Could you check a few things on this model? Use its own coordinates, in mm. Round coordinates to 2 decimals unless told otherwise and drop trailing zeros. Loops run counter-clockwise (first coordinate to the right, second up) from the corner with the lowest first, then second, coordinate; pieces in that order, holes last. Notation, with made-up numbers: M 89,-34.5 L 135,-34.5 A21 cw 135,-22.5 Z; hole C -38.5,-23 d11. An arc over 180 degrees is marked long. One line per item, written item: value. Start each with the question number.
Q1. Imagine slicing it at D-D (x = 30). Please give me the cut outline in (y, z), then the cut area to 3 significant figures.
Q2. Imagine slicing it at A-A (x = -8). Please give me the cut outline in (y, z), then the cut area to 3 significant figures.
Q3. I'm going to push flat-ended pins straight in: pin 1 Ø2 at (y, z) = (24, 3) entering from +X; pin 2 Ø8 at (x, y) = (14, -25) entering from +Z. Where does each tip first touch, or does it pass through?
Q4. Imagine slicing it at C-C (z = 2.05). Please give me the cut outline in (x, y).
Q5. Please list where these lines run through material, in increasing order: line 1 along Y through (x, z) = (-28, 3.65); line 2 along X through (y, z) = (45, 2.1); line 3 along Y through (x, z) = (-28.5, 0.6).
Q6. Imagine slicing it at B-B (y = -10). Please give me the cut outline in (x, z), then the cut area to 3 significant figures.
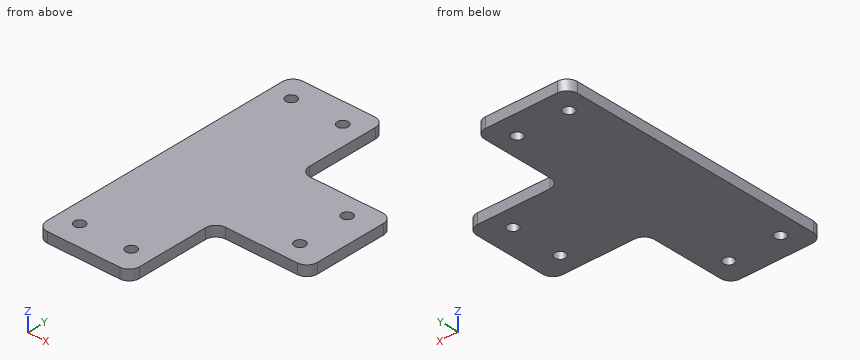
from build123d import *

# Parameters (mm, degrees)
BOSS_EXTRUDE1_DEPTH   = 4
M5X0_8_TAPPED_HOLE1_D = 4.2
FILLET1_R             = 4


with BuildPart() as part:
    # Sketch1 → Boss-Extrude1 (new body)
    with BuildSketch(Plane.XY):
        Polygon((0, -18), (0, -54), (-36, -54), (-36, 54), (0, 54), (0, 18), (36, 18), (36, -18), align=None)
    extrude(amount=BOSS_EXTRUDE1_DEPTH)

    # M5x0.8 Tapped Hole1 (through all)
    with Locations(Plane.XY.offset(4)):
        with Locations((-28, 44.91241041), (-8, 44.91241041), (25.616827634, 10), (25.616827634, -10), (-28, -44.758024198), (-8, -44.758024198)):
            Hole(M5X0_8_TAPPED_HOLE1_D / 2)

    # Fillet1
    fillet1_edges = [part.edges().sort_by_distance(p)[0] for p in [
        (-36, 54, 2),
        (0, 54, 2),
        (0, 18, 2),
        (36, 18, 2),
        (36, -18, 2),
        (0, -18, 2),
        (0, -54, 2),
        (-36, -54, 2),
    ]]
    fillet(fillet1_edges, radius=FILLET1_R)


solid = part.part
Report:
1. outline: M -18,0 L 18,0 L 18,4 L -18,4 Z
1. area: 144 mm²
2. outline: M -54,0 L -46.86,0 L -46.86,4 L -54,4 Z; M -42.66,0 L 42.81,0 L 42.81,4 L -42.66,4 Z; M 47.01,0 L 54,0 L 54,4 L 47.01,4 Z
2. area: 398 mm²
3. pin 1: stops at x = 0
3. pin 2: passes through
4. outline: M -36,-50 A4 ccw -32,-54 L -4,-54 A4 ccw 0,-50 L 0,-22 A4 cw 4,-18 L 32,-18 A4 ccw 36,-14 L 36,14 A4 ccw 32,18 L 4,18 A4 cw 0,22 L 0,50 A4 ccw -4,54 L -32,54 A4 ccw -36,50 Z; hole C -28,-44.76 d4.2; hole C -28,44.91 d4.2; hole C -8,-44.76 d4.2; hole C -8,44.91 d4.2; hole C 25.62,-10 d4.2; hole C 25.62,10 d4.2
5. line 1: y = -54 to -46.86, -42.66 to 42.81, 47.01 to 54
5. line 2: x = -36 to -30.1, -25.9 to -10.1, -5.9 to 0
5. line 3: y = -54 to -46.8, -42.72 to 42.87, 46.95 to 54
6. outline: M -36,0 L 23.52,0 L 23.52,4 L -36,4 Z; M 27.72,0 L 36,0 L 36,4 L 27.72,4 Z
6. area: 271 mm²
